Can you work these out from the drawing? Everything is in mm from the part's minimum corner. A direction names the side the tool comes from. Round coordinates to 2 decimals unless told otherwise and drop trailing zeros. Write each loop counter-clockwise with the first axis right and the second up, starting at its lowest first coordinate (ties: lowest second). Pieces come first, ordered by that corner, then holes.
Q1. If we section it at A-A (y = 8.5): Please give me the cut outline in (x, z).
Q2. If we section it at D-D (x = 14): Please give me the cut outline in (y, z).
Q3. For the marked faces 1, 2 and 3, which set-ups out of +Z, -Z, +X, -X, +Y, -Y let a thin tool reach every point of the face, with its end or its side?
Q4. I'm going to push flat-ended pins straight in: pin 1 Ø1.5 at (y, z) = (2.5, 7.5) entering from -X; pin 2 Ø3 at (y, z) = (12, 31.75) entering from -X; pin 3 Ø4 at (y, z) = (11, 3) entering from +X; pin 4 Ø3 at (x, y) = (18.5, 8) entering from +Z. Where does each tip first touch, or does it pass through?
Q5. If we section it at C-C (x = 28.75): Please give me the cut outline in (y, z).
Q6. Please list where these lines run through material, in increasing order: line 1 along Z through (x, y) = (6.25, 1.95); line 2 along X through (y, z) = (15.75, 32); line 3 along Z through (x, y) = (22, 16.25).
Q7. If we section it at B-B (z = 3.25): Please give me the cut outline in (x, y).
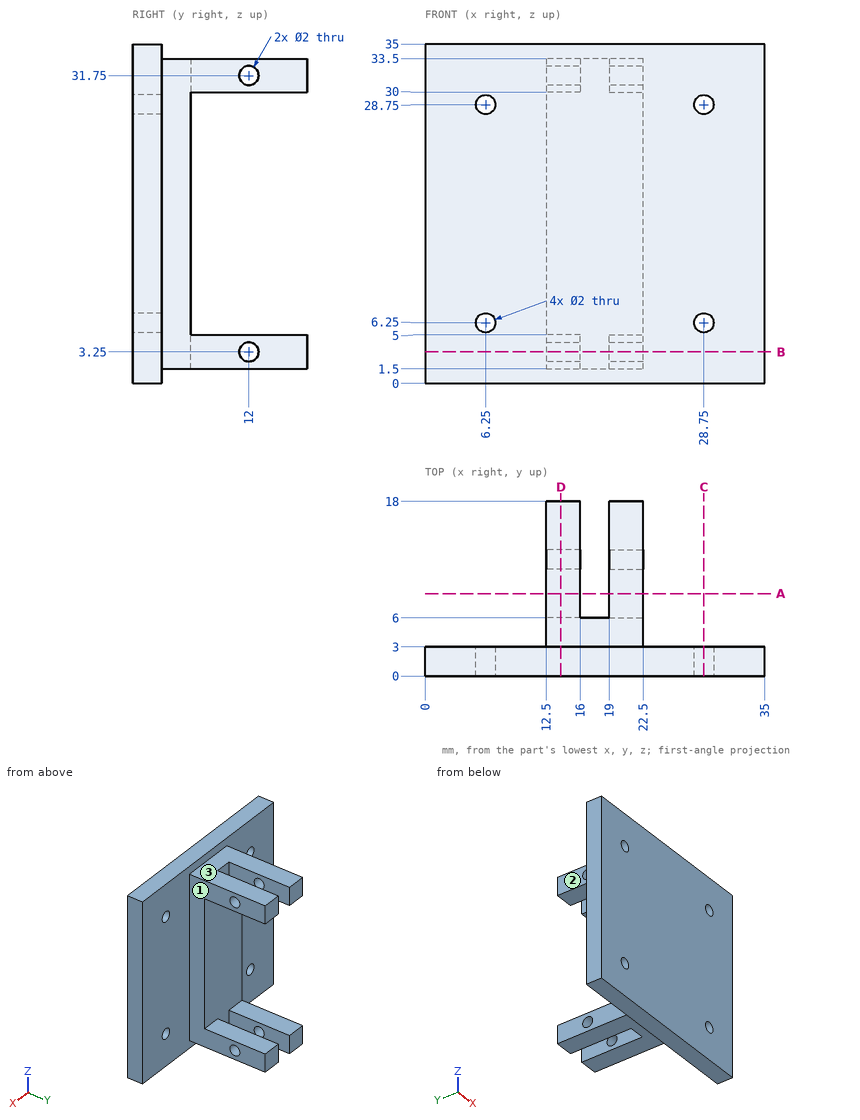
A:
1. outline: (12.5, 1.5) - (16, 1.5) - (16, 5) - (12.5, 5) - close; (12.5, 30) - (16, 30) - (16, 33.5) - (12.5, 33.5) - close; (19, 1.5) - (22.5, 1.5) - (22.5, 5) - (19, 5) - close; (19, 30) - (22.5, 30) - (22.5, 33.5) - (19, 33.5) - close
2. outline: (0, 0) - (3, 0) - (3, 1.5) - (18, 1.5) - (18, 5) - (6, 5) - (6, 30) - (18, 30) - (18, 33.5) - (3, 33.5) - (3, 35) - (0, 35) - close; hole circle Ø2 at (12, 3.25); hole circle Ø2 at (12, 31.75)
3. face 1: +Z, -Z, +X, +Y
3. face 2: +Z, -Z, -X, +Y
3. face 3: +Z, +X, -X, +Y
4. pin 1: stops at x = 0
4. pin 2: stops at x = 12.5
4. pin 3: stops at x = 22.5
4. pin 4: stops at z = 33.5
5. outline: (0, 0) - (3, 0) - (3, 5.25) - (0, 5.25) - close; (0, 7.25) - (3, 7.25) - (3, 27.75) - (0, 27.75) - close; (0, 29.75) - (3, 29.75) - (3, 35) - (0, 35) - close
6. line 1: z = 0 to 5.25, 7.25 to 27.75, 29.75 to 35
6. line 2: x = 12.5 to 16, 19 to 22.5
6. line 3: z = 1.5 to 5, 30 to 33.5
7. outline: (0, 0) - (35, 0) - (35, 3) - (22.5, 3) - (22.5, 11) - (19, 11) - (19, 6) - (16, 6) - (16, 11) - (12.5, 11) - (12.5, 3) - (0, 3) - close; (12.5, 13) - (16, 13) - (16, 18) - (12.5, 18) - close; (19, 13) - (22.5, 13) - (22.5, 18) - (19, 18) - close
